Here's how the part is built. I have some questions about the finished solid (model axes, mm). Give positions to 0.01 mm unless a question says otherwise; leave off trailing zeros. Write each loop counter-clockwise with the first axis right and the second up, starting at its lowest first coordinate (ties: lowest second). Pieces come first, ordered by that corner, then holes. Notation, with made-up numbers: (82.25, 10) -> (118.25, 10) arc R8 cw to (118.25, 25) -> close; hole circle Ø4 at (-30, 62.25). An arc over 180 degrees is marked (long way). Put each result on its own line as item: value. Start each with the question number.
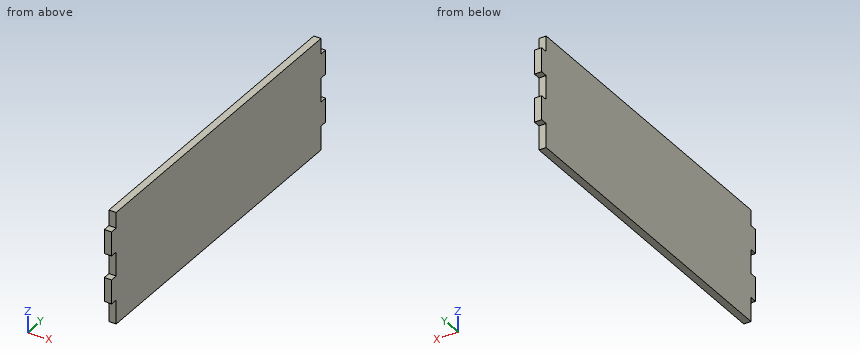
Autodesk Inventor part; units mm, degrees
ref_plane "YZ Plane" through (0, 0, 0) normal (1, 0, 0) x (0, 1, 0)
ref_plane "XZ Plane" through (0, 0, 0) normal (0, 1, 0) x (-1, 0, 0)
ref_plane "XY Plane" through (0, 0, 0) normal (0, 0, 1) x (1, 0, 0)
sketch "Sketch1" plane through (0, 0, 0) normal (0, 1, 0) x (-1, 0, 0)
  line L0 (0, 0) -> (0, -10)
  line L1 (0, -10) -> (3, -10)
  line L2 (0, 0) -> (0, 10)
  line L3 (0, 10) -> (0, 20)
  line L4 (0, 20) -> (0, 30)
  line L5 (0, 30) -> (0, 36.5)
  line L6 (0, 36.5) -> (3, 36.5)
  line L7 (3, 36.5) -> (3, -10)
  line L8 (3, 30) -> (0, 30)
  line L9 (0, 20) -> (3, 20)
  line L10 (0, 10) -> (3, 10)
  line L11 (0, 0) -> (3, 0)
  dimension "d0" = 10
  dimension "d1" = 3
  dimension "d2" = 10
  dimension "d3" = 10
  dimension "d4" = 10
  dimension "d5" = 6.5
  dimension "d6" = 3
extrude "Extrusion1" add sketch "Sketch1" along normal blind 3 contours L2 L10 L7 L11 | L4 L8 L7 L9
sketch "Sketch2" plane through (0, 3, 0) normal (0, 1, 0) x (1, 0, 0)
  line L0 (0, 0) -> (0, 10)
  line L1 (-3, -20) -> (-3, -30)
  line L2 (0, 10) -> (-3, 10)
  line L3 (-3, 10) -> (-3, -30)
  line L4 (-3, -30) -> (0, -30)
  line L5 (0, -30) -> (0, 10)
  line L6 (0, -30) -> (0, -36.5)
  line L7 (0, -36.5) -> (-3, -36.5)
  line L8 (-3, -36.5) -> (-3, -30)
  line L9 (-3, -30) -> (0, -30)
  line L10 (0, -30) -> (0, -36.5)
  dimension "d9" = 10
  dimension "d10" = 6.5
extrude "Extrusion2" add sketch "Sketch2" along normal blind 67
mirror "Mirror1" about plane through (-1.5, 70, 13.25) normal (0, 1, 0) of "Extrusion2", "Extrusion1"
properties part number "motorkap"
1) I want a section at B-B, the plane z = -2.5. Write out the boundary of the cut face in (x, y), and give its area (3 significant figures).
2) I need wall thicknesses on probe 1 along Y at (x, z) = (-1.25, 12.5). Which ranges of the line are inside material? Lowest first, please.
3) I want a section at A-A, the plane x = -1.65. Write out the boundary of the cut face in (y, z).
4) I'm going to push flat-ended pins straight in: pin 1 Ø0.9 at (x, y) = (-2, 1) entering from +Z; pin 2 Ø1.5 at (x, z) = (-1, -3) entering from -Y; pin 3 Ø1.5 at (x, z) = (-1, 16) entering from +Y. Where does each tip first touch, or does it pass through?
Established:
1. outline: (-3, 3) -> (0, 3) -> (0, 137) -> (-3, 137) -> close
1. area: 402 mm2
2. probe 1: y = 3 to 137
3. outline: (0, 0) -> (3, 0) -> (3, -10) -> (137, -10) -> (137, 0) -> (140, 0) -> (140, 10) -> (137, 10) -> (137, 20) -> (140, 20) -> (140, 30) -> (137, 30) -> (137, 36.5) -> (3, 36.5) -> (3, 30) -> (0, 30) -> (0, 20) -> (3, 20) -> (3, 10) -> (0, 10) -> close
4. pin 1: stops at z = 30
4. pin 2: stops at y = 3
4. pin 3: stops at y = 137
